Model file for the job. Use its own axes, mm. Give positions to 0.01 mm unless a question says otherwise; leave off trailing zeros. Loops run counter-clockwise (first coordinate to the right, second up) from the corner with the lowest first, then second, coordinate; pieces in that order, holes last. Notation, with made-up numbers: (48, -12) - (53, -12) arc R13 ccw to (53, 7) - close; hole circle Ø11 at (40.5, 63.5). An arc over 180 degrees is marked (long way). Use a Markdown table: item, result.
from build123d import *

# Parameters (mm, degrees)
BOSS_EXTRUDE1_DEPTH = 10
SKETCH2_R           = 10
CUT_EXTRUDE1_DEPTH  = 10
CUT_EXTRUDE3_DEPTH  = 4


with BuildPart() as part:
    # Sketch1 → Boss-Extrude1 (new body)
    with BuildSketch(Plane(origin=(0, 0, 0), x_dir=(1, 0, 0), z_dir=(0, 1, 0))):
        Polygon((60, -60), (60, -180), (-60, -180), (-60, -60), (-180, -60), (-180, 60), (-60, 60), (-60, 180), (60, 180), (60, 60), (180, 60), (180, -60), align=None)
        with BuildLine():
            Line((-60, 180), (-60, 60))
            Line((-60, 60), (-180, 60))
            ThreePointArc((-180, 60), (-95.147186258, 95.147186258), (-60, 180))
        make_face()
        with BuildLine():
            ThreePointArc((60, 180), (95.147186258, 95.147186258), (180, 60))
            Line((180, 60), (60, 60))
            Line((60, 60), (60, 180))
        make_face()
        with BuildLine():
            ThreePointArc((180, -60), (95.147186258, -95.147186258), (60, -180))
            Line((60, -180), (60, -60))
            Line((60, -60), (180, -60))
        make_face()
        with BuildLine():
            Line((-180, -60), (-60, -60))
            Line((-60, -60), (-60, -180))
            ThreePointArc((-60, -180), (-95.147186258, -95.147186258), (-180, -60))
        make_face()
    extrude(amount=BOSS_EXTRUDE1_DEPTH)

    # Sketch2 → Cut-Extrude1 (cut)
    with BuildSketch(Plane.XZ):
        with Locations((0, -90)):
            Circle(SKETCH2_R)
    extrude(amount=-CUT_EXTRUDE1_DEPTH, mode=Mode.SUBTRACT)

    # Sketch5 → Cut-Extrude3 (cut)
    with BuildSketch(Plane.XZ):
        Polygon((24.5, -110), (-24.5, -110), (-28.5, -110), (-28.5, -114), (28.5, -114), (28.5, -110), align=None)
    extrude(amount=-CUT_EXTRUDE3_DEPTH, mode=Mode.SUBTRACT)


solid = part.part
(1) Slice it at C-C, the plane z = -90. Write the cut outline in (x, y), plus the area to 3 significant figures.
Computed:
| item | result |
|---|---|
| outline | (-100.63, 0) - (-10, 0) - (-10, 10) - (-100.63, 10) - close; (10, 0) - (100.63, 0) - (100.63, 10) - (10, 10) - close |
| area | 1,810 mm² |
(2) Mould opens along X. For faces 1 (the cylindrical face through (-96.085, 4.93, -94.219)), 2 (the cylindrical face through (96.085, 4.93, 94.219)), 3 (the cylindrical face through (-1.302, 4.93, -80.085)) say: pulls with the +X half, pulls with the -X half, needs draft (parallel to the pull), parting line crosses it, or undercut.
Computed:
| item | result |
|---|---|
| face 1 | pulls with the -X half |
| face 2 | pulls with the +X half |
| face 3 | undercut |
(3) Slice it at D-D, the plane x = 118. Write the cut outline in (y, z), plus the area to 3 significant figures.
Computed:
| item | result |
|---|---|
| outline | (0, -77.26) - (10, -77.26) - (10, 77.26) - (0, 77.26) - close |
| area | 1,550 mm² |
(4) Drill centre lines: probe 1 along Z at (x, y) = (0, 2.5); probe 2 along Z at (x, y) = (6.5, 3); probe 3 along Z at (x, y) = (0, 5). Where is each one in solid material? Low to high. Write a range as [from, to].
Computed:
| item | result |
|---|---|
| probe 1 | [-180, -114], [-110, -100], [-80, 180] |
| probe 2 | [-180, -114], [-110, -97.6], [-82.4, 180] |
| probe 3 | [-180, -100], [-80, 180] |
(5) Slice it at A-A, the plane y = 6.25. Write the cut outline in (x, z), plus the area to 3 significant figures.
Computed:
| item | result |
|---|---|
| outline | (-180, -60) arc R120 cw to (-60, -180) - (60, -180) arc R120 cw to (180, -60) - (180, 60) arc R120 cw to (60, 180) - (-60, 180) arc R120 cw to (-180, 60) - close; hole circle Ø20 at (0, -90) |
| area | 84,000 mm² |
(6) Pin check, flat tips, straight feed: P1, Ø3, axis at y = 3.5, z = -104, coming from the +X side; P2, Ø3, axis at y = 3, z = -111, coming from the +X side; P3, Ø6, axis at y = 7, z = 109.5, coming from the -X side. Stop position of each tip, or through.
Computed:
| item | result |
|---|---|
| P1 | x = 88.38 |
| P2 | x = 82.89 |
| P3 | x = -85.14 |
(7) Slice it at B-B, the plane x = 0. Write the cut outline in (y, z).
Computed:
| item | result |
|---|---|
| outline | (0, -180) - (10, -180) - (10, -100) - (0, -100) - (0, -110) - (4, -110) - (4, -114) - (0, -114) - close; (0, -80) - (10, -80) - (10, 180) - (0, 180) - close |
